Model file for the job. Use its own axes, mm. Face numbers are marked on the shaded views. A direction names the side the tool comes from. Round coordinates to 2 decimals unless told otherwise and drop trailing zeros. Order: outer loops, then holes, each group sorted by start corner. A loop starts at its lowest first (then second) coordinate and runs counter-clockwise, first axis right, second up. Notation, with made-up numbers: (64, -12.75) -> (82, -12.75) arc R17 ccw to (82, -4.75) -> close; hole circle Ø1 at (16.5, -6.75). An arc over 180 degrees is marked (long way). Put each result on its own line as item: value. Start each with the question number.
Q1. Pull direction Y, two halves, no side cores. Call the marked faces 1, 2 and 3: released by +Y, released by -Y, zero draft, split by the parting line, or undercut.
Q2. Cut at B-B, the plane x = -10. List the corners of the cut face in (y, z), and give its area (3 significant figures).
Q3. Flat gauge pins, fed straight in: P1, Ø5, axis at x = 47.5, z = -14.5, coming from the -Y side; P2, Ø3, axis at y = 13.5, z = -20, coming from the -X side; P3, Ø6, axis at x = 1, y = 12.5, coming from the -Z side. Where does each tip first touch, or does it go through?
Q4. 3-axis set-ups, long thin cutter, end or side, ignore diameter. For the marked faces 4 and 5: which of +Z, -Z, +X, -X, +Y, -Y reach the whole face in a straight line?
Q5. Probe L1, parallel to Z at x = 52, y = -4.5; L2, parallel to X at y = -13.5, z = -37; L3, parallel to X at y = 19, z = -35.5. List the from-to ranges inside material, lowest first.
Q6. Cut at C-C, the plane y = 2. List the corners of the cut face in (x, z), and give its area (3 significant figures).
Q7. Cut at A-A, the plane y = 16. List the corners of the cut face in (x, z).
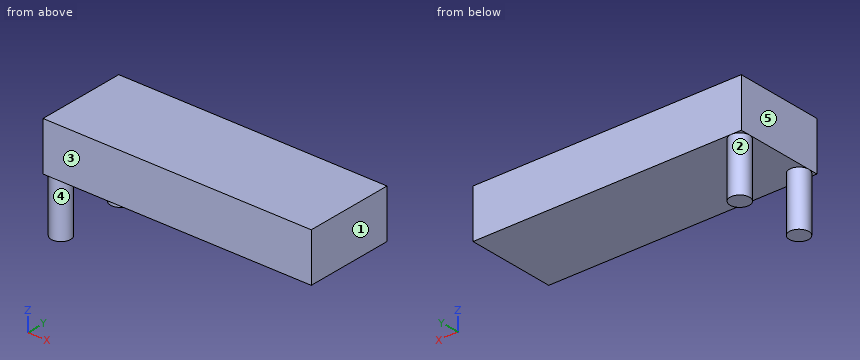
Autodesk Inventor part; units mm, degrees
ref_plane "YZ Plane" through (0, 0, 0) normal (1, 0, 0) x (0, 1, 0)
ref_plane "XZ Plane" through (0, 0, 0) normal (0, 1, 0) x (-1, 0, 0)
ref_plane "XY Plane" through (0, 0, 0) normal (0, 0, 1) x (1, 0, 0)
sketch "Szkic1" plane through (0, 0, 0) normal (0, 0, 1) x (1, 0, 0)
  line L0 (-69, -23) -> (69, -23)
  line L1 (69, -23) -> (69, 23)
  line L2 (69, 23) -> (-69, 23)
  line L3 (-69, 23) -> (-69, -23)
  line L4 (-69, -23) -> (69, 23) construction
  line L5 (69, -23) -> (-69, 23) construction
  point P0 (0, 0)
  dimension "d0" = 138
  dimension "d1" = 46
extrude "Wyciągnięcie proste1" add sketch "Szkic1" along normal mid plane 25
sketch "Szkic2" plane through (0, 0, -12.5) normal (0, 0, -1) x (-1, 0, 0)
  line L0 (-69, -23) -> (69, -23)
  line L1 (69, -23) -> (69, 23)
  line L2 (69, 23) -> (-69, 23)
  line L3 (-69, 23) -> (-69, -23)
  circle A0 centre (64, -18) radius 5
  circle A1 centre (64, 18) radius 5
  line L4 (-69, -23) -> (69, -23)
  line L5 (69, -23) -> (69, 23)
  line L6 (69, 23) -> (-69, 23)
  point P0 (0, 0)
  dimension "d4" = 10
  dimension "d5" = 10
extrude "Wyciągnięcie proste2" add sketch "Szkic2" along normal blind 28 contours A0 | A1
equation "\"d5\" = d4"
properties part number "lipol_6000"
Ans:
1. face 1: zero draft
1. face 2: undercut
1. face 3: released by -Y
2. outline: (-23, -12.5) -> (23, -12.5) -> (23, 12.5) -> (-23, 12.5) -> close
2. area: 1,150 mm^2
3. P1: stops at y = -23
3. P2: stops at x = -68
3. P3: stops at z = -12.5
4. face 4: -Z
4. face 5: +Z, -Z, -X, +Y, -Y
5. L1: z = -12.5 to 12.5
5. L2: x = -66.18 to -61.82
5. L3: x = -68.9 to -59.1
6. outline: (-69, -12.5) -> (69, -12.5) -> (69, 12.5) -> (-69, 12.5) -> close
6. area: 3,450 mm^2
7. outline: (-69, -12.5) -> (-68.58, -12.5) -> (-68.58, -40.5) -> (-59.42, -40.5) -> (-59.42, -12.5) -> (69, -12.5) -> (69, 12.5) -> (-69, 12.5) -> close
